from build123d import *

# Parameters (mm, degrees)
F1_DEPTH = 1246
F2_R     = 25
F3_DEPTH = 5
F4_R     = 7
F5_DEPTH = 305.001


with BuildPart() as f1:
    # F0 (on Front) → F1 (new body)
    with BuildSketch(Plane.XZ):
        with BuildLine():
            Line((0, 5), (0, 0))
            Line((0, 0), (62, 0))
            ThreePointArc((62, 0), (72.606602, 4.393398), (77, 15))
            Line((77, 15), (77, 290))
            ThreePointArc((77, 290), (72.606602, 300.606602), (62, 305))
            Line((62, 305), (0, 305))
            Line((0, 305), (0, 300))
            Line((0, 300), (62, 300))
            ThreePointArc((62, 300), (69.071068, 297.071068), (72, 290))
            Line((72, 290), (72, 15))
            ThreePointArc((72, 15), (69.071068, 7.928932), (62, 5))
            Line((62, 5), (0, 5))
        make_face()
    extrude(amount=F1_DEPTH)

    # F2 (on face) → F3 (cut, through all)
    with BuildSketch(Plane.YZ.offset(77)):
        with Locations((-623, 190)):
            Circle(F2_R)
    extrude(amount=-F3_DEPTH, mode=Mode.SUBTRACT)

    # F4 (on face) → F5 (cut, through all)
    with BuildSketch(Plane.XY.offset(305)):
        with Locations((38, -1155)):
            Circle(F4_R)
        with Locations((38, -1003)):
            Circle(F4_R)
        with Locations((38, -851)):
            Circle(F4_R)
        with BuildLine():
            ThreePointArc((45, -699), (38, -692), (31, -699))
            ThreePointArc((31, -699), (38, -706), (45, -699))
        make_face()
        with Locations((38, -547)):
            Circle(F4_R)
        with Locations((38, -395)):
            Circle(F4_R)
        with Locations((38, -243)):
            Circle(F4_R)
        with Locations((38, -91)):
            Circle(F4_R)
    extrude(amount=-F5_DEPTH, mode=Mode.SUBTRACT)


solid = f1.part
Geometry check sheet. Reference: the model listing, model coordinates, mm. A direction names the side the tool comes from. Round coordinates to 2 decimals unless told otherwise and drop trailing zeros. Write each loop counter-clockwise with the first axis right and the second up, starting at its lowest first coordinate (ties: lowest second). Pieces come first, ordered by that corner, then holes. Notation, with made-up numbers: (34.5, 10.25) - (78.5, 10.25) arc R18 cw to (78.5, 16.25) - close; hole circle Ø7 at (-28, 11). An arc over 180 degrees is marked (long way). One line per item, written item: value.
1. Depth check by flat-ended pin: pin 1 Ø10 at (y, z) = (-923.5, 137.5) entering from -X. Enter the tip coordinate at first touch or a pass-through.
The answers:
pin 1: stops at x = 72
2. Set-up check for faces 1 (the face through (31, -614, 5)), 2 (the face through (73, 0, 198)): record each of +Z, -Z, +X, -X, +Y, -Y from which the full face is reachable in a straight line by a thin tool's end or side.
The answers:
face 1: -X, +Y, -Y
face 2: +Z, -Z, +X, -X, +Y
3. Cross-section at A-A on y = -1106. Record the boundary of the cut face in (x, z), and give its area (3 significant figures).
The answers:
outline: (0, 0) - (62, 0) arc R15 ccw to (77, 15) - (77, 290) arc R15 ccw to (62, 305) - (0, 305) - (0, 300) - (62, 300) arc R10 cw to (72, 290) - (72, 15) arc R10 cw to (62, 5) - (0, 5) - close
area: 2,190 mm^2
4. Scan lines: L1, parallel to Z at x = 22, y = -777; L2, parallel to Z at x = 64, y = -458; L3, parallel to X at y = -851, z = 3.8. Record each from-to range of solid material in increasing order.
The answers:
L1: z = 0 to 5, 300 to 305
L2: z = 0.13 to 5.2, 299.8 to 304.87
L3: x = 0 to 31, 45 to 71.98
5. Mould release check, pull along Z, two halves, no side actions. Record for faces 3 (the face through (31, -614, 0)), 4 (the face through (31, -614, 305)), 5 (the face through (31, -614, 300)), 6 (the face through (73, -1246, 198)): released by +Z, released by -Z, zero draft, split by the parting line, or undercut.
The answers:
face 3: released by -Z
face 4: released by +Z
face 5: undercut
face 6: zero draft
6. Cross-section at B-B on z = 230. Record the boundary of the cut face in (x, y), and give its area (3 significant figures).
The answers:
outline: (72, -1246) - (77, -1246) - (77, 0) - (72, 0) - close
area: 6,230 mm^2
